Could you check a few things on this model? Use its own coordinates, in mm. Face numbers are marked on the shaded views. A direction names the side the tool comes from. Coordinates: 2 decimals unless noted, no trailing zeros. Loops run counter-clockwise (first coordinate to the right, second up) from the corner with the lowest first, then second, coordinate; pieces in that order, holes last. Notation, with made-up numbers: (-31, 52.25) - (-27, 52.25) arc R21 cw to (-27, 56.25) - close; hole circle Ø4 at (38.25, 89). An arc over 180 degrees is marked (long way). Put each result on its own line as item: value. Start each with the question number.
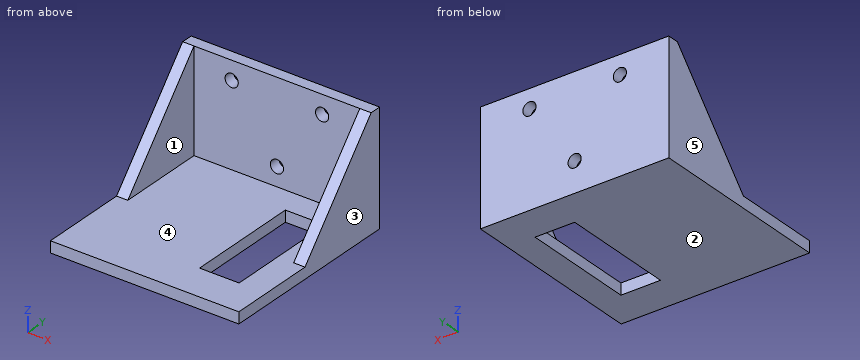
```python
from build123d import *

# Parameters (mm, degrees)
F0_W     = 50
F0_H     = 3
F1_DEPTH = 30
F0_H_2   = 47
F0_W_2   = 10.5
F0_H_3   = 30.5
F2_DEPTH = 3
F4_DEPTH = 3
F6_DEPTH = 3
F7_R     = 1.75
F8_DEPTH = 3


with BuildPart() as f1:
    # F0 (on Top) → F1 (new body)
    with BuildSketch(Plane.XY):
        with Locations((-17.8984425962, 25.9814620614)):
            Rectangle(F0_W, F0_H)
    extrude(amount=F1_DEPTH)

    # F0 (on Top) → F2 (join)
    with BuildSketch(Plane.XY):
        with Locations((-17.8984425962, 0.9814620614)):
            Rectangle(F0_W, F0_H_2)
        with Locations((-30.4321678579, 2.4814620614)):
            Rectangle(F0_W_2, F0_H_3, mode=Mode.SUBTRACT)
        with Locations((-5.3647173345, 2.4814620614)):
            Rectangle(F0_W_2, F0_H_3, mode=Mode.SUBTRACT)
        with Locations((-30.4321678579, 2.4814620614)):
            Rectangle(F0_W_2, F0_H_3)
    extrude(amount=F2_DEPTH)

    # F3 (on face) → F4 (join)
    with BuildSketch(Plane(origin=(-42.8984425962, 0, 0), x_dir=(0, -1, 0), z_dir=(-1, 0, 0))):
        Polygon((-0.9814620614, 3), (-24.4814620614, 30), (-24.4814620614, 3), align=None)
    extrude(amount=-F4_DEPTH)

    # F5 (on face) → F6 (join)
    with BuildSketch(Plane.YZ.offset(7.1015574038)):
        Polygon((24.4814620614, 3), (24.4814620614, 30), (0.9814620614, 3), align=None)
    extrude(amount=-F6_DEPTH)

    # F7 (on face) → F8 (cut)
    with BuildSketch(Plane.XZ.offset(-24.4814620614)):
        with Locations((-29.8984425962, 25)):
            Circle(F7_R)
        with Locations((-5.8984425962, 25)):
            Circle(F7_R)
        with Locations((-17.8984425962, 8)):
            Circle(F7_R)
    extrude(amount=-F8_DEPTH, mode=Mode.SUBTRACT)


solid = f1.part
```
(1) I want a section at D-D on z = 8. List the corners of the cut face in (x, y) for me.
(2) For pin 1 Ø4 at (x, z) = (-5.9, 25) entering from +Y; pin 2 Ø2 at (x, z) = (-17.9, 8) entering from -Y; pin 3 Ø6 at (x, y) = (-3, 20) entering from +Z; pin 4 Ø8 at (x, z) = (-24.5, 14.5) entering from -Y, each with a flat end and sliding along its axis, tell me the tip position at first contact or that it passes through.
(3) Which directions (+Z, -Z, +X, -X, +Y, -Y) give clear straight access to the entire face, cutting with the end or side of a thin tool? Please do the marked faces 1 and 2.
(4) If we mould it in two halves opening along X, with no side actions, what happens to the marked faces 3, 4 and 5? For each: pulls with the +X half, pulls with the -X half, needs draft (parallel to the pull), parting line crosses it, or undercut.
(5) I want a section at A-A on y = -11. List the corners of the cut face in (x, z) for me, and give its area (4 significant figures).
(6) I want a section at C-C on x = -30.5. List the corners of the cut face in (y, z) for me.
(7) I need wall thicknesses on L1, parallel to X at y = 20, z = 8; L2, parallel to Y at x = -22, z = 3.25; L3, parallel to Z at x = -36.5, y = -3.5. Which ranges of each line are inside material? Lowest first, please. Write a range as [from, to].
(8) I want a section at B-B on z = 25. List the corners of the cut face in (x, y) for me, and give its area (3 significant figures).
Answer sheet:
1. outline: (-42.9, 5.33) - (-39.9, 5.33) - (-39.9, 24.48) - (-19.65, 24.48) - (-19.65, 27.48) - (-42.9, 27.48) - close; (-16.15, 24.48) - (4.1, 24.48) - (4.1, 5.33) - (7.1, 5.33) - (7.1, 27.48) - (-16.15, 27.48) - close
2. pin 1: stops at y = 27.48
2. pin 2: passes through
2. pin 3: stops at z = 3
2. pin 4: stops at y = 24.48
3. face 1: +Z, -Y
3. face 2: -Z, +X, -X, +Y, -Y
4. face 3: pulls with the +X half
4. face 4: undercut
4. face 5: pulls with the -X half
5. outline: (-42.9, 0) - (-10.61, 0) - (-10.61, 3) - (-42.9, 3) - close; (-0.11, 0) - (7.1, 0) - (7.1, 3) - (-0.11, 3) - close
5. area: 118.5 mm^2
6. outline: (-22.52, 0) - (27.48, 0) - (27.48, 23.36) - (24.48, 23.36) - (24.48, 3) - (-22.52, 3) - close; (24.48, 26.64) - (27.48, 26.64) - (27.48, 30) - (24.48, 30) - close
7. L1: x = [-42.9, -39.9], [4.1, 7.1]
7. L2: y = [24.48, 27.48]
7. L3: z = [0, 3]
8. outline: (-42.9, 20.13) - (-39.9, 20.13) - (-39.9, 24.48) - (-31.65, 24.48) - (-31.65, 27.48) - (-42.9, 27.48) - close; (-28.15, 24.48) - (-7.65, 24.48) - (-7.65, 27.48) - (-28.15, 27.48) - close; (-4.15, 24.48) - (4.1, 24.48) - (4.1, 20.13) - (7.1, 20.13) - (7.1, 27.48) - (-4.15, 27.48) - close
8. area: 155 mm^2
